Autodesk Inventor part; units mm, degrees
ref_plane "YZ Plane" through (0, 0, 0) normal (1, 0, 0) x (0, 1, 0)
ref_plane "XZ Plane" through (0, 0, 0) normal (0, 1, 0) x (-1, 0, 0)
ref_plane "XY Plane" through (0, 0, 0) normal (0, 0, 1) x (1, 0, 0)
sketch "Sketch1" plane through (0, 0, 0) normal (0, 1, 0) x (-1, 0, 0)
  line L0 (-7, 7) -> (7, 7)
  line L1 (7, 7) -> (7, -7)
  line L2 (7, -7) -> (-7, -7)
  line L3 (-7, -7) -> (-7, 7)
  line L4 (-7, 7) -> (7, -7) construction
  line L5 (7, 7) -> (-7, -7) construction
  point P0 (0, 0)
  dimension "d0" = 14
  dimension "d1" = 14
extrude "Extrusion1" add sketch "Sketch1" along normal blind 4
sketch "Sketch2" plane through (0, 4, 0) normal (0, 1, 0) x (1, 0, 0)
  line L0 (8, 8) -> (-8, 8)
  line L1 (-8, 8) -> (-8, -8)
  line L2 (-8, -8) -> (8, -8)
  line L3 (8, -8) -> (8, 8)
  line L4 (8, 8) -> (-8, -8) construction
  line L5 (-8, 8) -> (8, -8) construction
  point P0 (0, 0)
  dimension "d4" = 16
  dimension "d5" = 16
extrude "Extrusion2" add sketch "Sketch2" along normal blind 0.6
sketch "Sketch3" plane through (0, 4.6, 0) normal (0, 1, 0) x (1, 0, 0)
  line L0 (3, -5.5611) -> (-5, -5.5611)
  line L1 (-5, -5.5611) -> (-5, 5.4389)
  line L2 (-5, 5.4389) -> (3, 5.4389)
  line L3 (3, 5.4389) -> (3, -5.5611)
  line L4 (3, -5.5611) -> (-5, 5.4389) construction
  line L5 (-5, -5.5611) -> (3, 5.4389) construction
  point P0 (0, 0)
  point P1 (-1, -0.0611)
  dimension "d8" = 8
  dimension "d9" = 11
extrude "Extrusion3" add sketch "Sketch3" along normal blind 6
sketch "Sketch4" plane through (0, 10.6, 0) normal (0, 1, 0) x (1, 0, 0)
  line L0 (8, -8) -> (-8, -8)
  line L1 (-8, -8) -> (-8, 8)
  line L2 (-8, 8) -> (8, 8)
  line L3 (8, 8) -> (8, -8)
  line L4 (8, -8) -> (-8, 8) construction
  line L5 (-8, -8) -> (8, 8) construction
  point P0 (0, 0)
  dimension "d12" = 16
  dimension "d13" = 16
extrude "Extrusion4" add sketch "Sketch4" along normal blind 7
chamfer "Chamfer1" distance 1 distance2 7 4 edges at (8, 17.6, 0) (0, 17.6, 8) (0, 17.6, -8) (-8, 17.6, 0) measured on face at (-2.6667, 17.6, 2.6667)
sketch "Sketch5" plane through (0, 0, 0) normal (0, -1, 0) x (1, 0, 0)
  circle A0 centre (0, 0) radius 2
  line L0 (-5, -5.4389) -> (3, -5.4389) construction
  line L1 (0, 0) -> (0, -11)
  line L2 (0, 0) -> (4.5527, 0)
  circle A1 centre (0, -5.5) radius 0.75
  circle A2 centre (0, 5.5) radius 0.75
  dimension "d19" = 4
  dimension "d22" = 1.5
  dimension "d23" = 5.5
extrude "Extrusion5" add sketch "Sketch5" along normal blind 3
chamfer "Chamfer2" distance 0.7 angle 45 3 edges at (-2, -3, 0) (-0.75, -3, 5.5) (-0.75, -3, -5.5)
properties part number "switch"
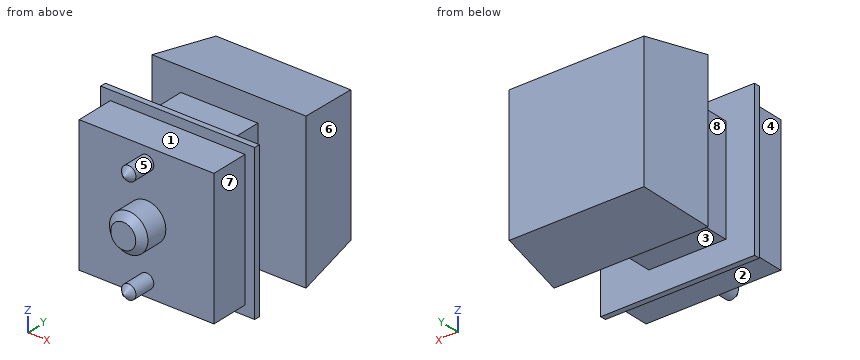
Here's how the part is built. I have some questions about the finished solid (model axes, mm). Face numbers are marked on the shaded views. A direction names the side the tool comes from. Coordinates: 2 decimals unless noted, no trailing zeros. Order: outer loops, then holes, each group sorted by start corner. A loop starts at its lowest first (then second) coordinate and runs counter-clockwise, first axis right, second up. Notation, with made-up numbers: (-20.75, 73.25) - (-7.75, 73.25) arc R12 ccw to (-7.75, 92.25) - close; hole circle Ø8 at (49.25, 31.5). An arc over 180 degrees is marked (long way). One line per question, with ' | ' between items. Start each with the question number.
1. Please list where these lines run through material, in increasing order: line 1 along Y through (x, z) = (3, 6); line 2 along Z through (x, y) = (-0.5, -1.25); line 3 along X through (y, z) = (5.25, -0.75). Write a range as [from, to].
2. If we section it at C-C (y = 8): Write out the boundary of the cut face in (x, z).
3. If we mould it in two halves opening along Y, with no side actions, what happens to the marked faces 6, 7 and 8? For each: released by +Y, released by -Y, zero draft, split by the parting line, or undercut.
4. I'm going to push flat-ended pins straight in: pin 1 Ø3 at (x, y) = (-1.5, 8.5) entering from -Z; pin 2 Ø6 at (y, z) = (12.5, -4.5) entering from -X; pin 3 Ø4.5 at (x, y) = (-1.5, 1.5) entering from +Z. Where does each tip first touch, or does it pass through?
5. Which directions (+Z, -Z, +X, -X, +Y, -Y) give clear straight access to the entire face, cutting with the end or side of a thin tool? Please do the marked faces 1, 2, 3, 4 and 5.
Model answer:
1) line 1: y = [0, 4.6], [10.6, 17.6] | line 2: z = [-6.06, -4.94], [-1.94, 1.94], [4.94, 6.06] | line 3: x = [-5, 3]
2) outline: (-5, -5.44) - (3, -5.44) - (3, 5.56) - (-5, 5.56) - close
3) face 6: released by +Y | face 7: zero draft | face 8: undercut
4) pin 1: stops at z = -5.44 | pin 2: stops at x = -8 | pin 3: stops at z = 7
5) face 1: +Z, +X, -X, -Y | face 2: -Z, +X, -X, -Y | face 3: -Z, +X, -X | face 4: +Z, -Z, -X, -Y | face 5: -Y
